Can you work these out from the model? Positions are in its coordinate system, mm. A direction names the side the tool comes from. Give positions to 0.01 mm unless a question says otherwise; leave off trailing zeros. Write each loop counter-clockwise with the first axis right and the second up, starting at its lowest first coordinate (ties: lowest second). Pieces come first, ordered by that corner, then holes. Notation, with made-up numbers: M 26,69.25 L 65,69.25 A20 cw 65,86.25 Z; hole C -7.5,38 d11. An arc over 180 degrees is marked long. Use CSV: the item, a comma, the result in double quotes. Start each with the question number.
from build123d import *

# Parameters (mm, degrees)
F1_DEPTH = 30
F3_D     = 3.5
F3_DEPTH = 5


with BuildPart() as f1:
    # F0 (on Front) → F1 (new body)
    with BuildSketch(Plane.XZ):
        Polygon((27.040993, 7.364779), (-2.959007, 7.364779), (-2.959007, -17.635221), (7.234091, -26.008121), (8.50357, -24.462669), (-0.959007, -16.689839), (-0.959007, 5.364779), (27.040993, 5.364779), align=None)
    extrude(amount=F1_DEPTH)

    # F3
    with Locations(Plane.XY.offset(7.364779)):
        with Locations((7.040993, -10), (17.040993, -15), (7.040993, -20)):
            Hole(F3_D / 2, depth=F3_DEPTH)


solid = f1.part
(1) I want a section at A-A (y = -20). Write out the boundary of the cut face in (x, z), and give its area (3 significant figures).
(2) Thinking about a two-plate mould opening in Y: for faces 4 (the face through (12, -15, 7.365)), 5 (the face through (-1.4, 0, -3.1)), 6 (the face through (-1.4, -30, -3.1)), 7 (the face through (7.269, -18.265, 6.351)), which applies, released by +Y, released by -Y, zero draft, split by the parting line, or undercut?
(3) I want a section at D-D (x = 22.5). Write out the boundary of the cut face in (y, z).
(4) Will these pins go through, and if not, where does the flat tip stop? pin 1 Ø6.5 at (y, z) = (-7.5, -8) entering from +X; pin 2 Ø5.5 at (x, y) = (17.04, -15) entering from -Z; pin 3 Ø10 at (x, z) = (9, -9) entering from -Y; pin 4 Ø4 at (x, y) = (9.5, -21.5) entering from -Z.
(5) I want a section at B-B (x = 17). Write out the boundary of the cut face in (y, z).
(6) Please list where these lines run through material, in increasing order: L1, parallel to Z at x = 19.75, y = -9.25; L2, parallel to X at y = -9.5, z = 3.5; L3, parallel to Z at x = -0.5, y = -13.75. Write a range as [from, to].
(7) Which directions (+Z, -Z, +X, -X, +Y, -Y) give clear straight access to the entire face, cutting with the end or side of a thin tool? Please do faces 1 (the face through (-0.959, -15, -6)), 2 (the face through (7.9, -14.8, -25.2)), 3 (the face through (7.269, -8.265, 6.351)).
(8) I want a section at C-C (y = -6.5). Write out the boundary of the cut face in (x, z), and give its area (3 significant figures).
Geometry results:
1,outline,"M -2.96,-17.64 L 7.23,-26.01 L 8.5,-24.46 L -0.96,-16.69 L -0.96,5.36 L 5.29,5.36 L 5.29,7.36 L -2.96,7.36 Z; M 8.79,5.36 L 27.04,5.36 L 27.04,7.36 L 8.79,7.36 Z"
1,area,"123 mm2"
2,face 4,"zero draft"
2,face 5,"released by +Y"
2,face 6,"released by -Y"
2,face 7,"undercut"
3,outline,"M -30,5.36 L 0,5.36 L 0,7.36 L -30,7.36 Z"
4,pin 1,"stops at x = -0.96"
4,pin 2,"stops at z = 5.36"
4,pin 3,"passes through"
4,pin 4,"stops at z = -25.68"
5,outline,"M -30,5.36 L -16.75,5.36 L -16.75,7.36 L -30,7.36 Z; M -13.25,5.36 L 0,5.36 L 0,7.36 L -13.25,7.36 Z"
6,L1,"z = [5.36, 7.36]"
6,L2,"x = [-2.96, -0.96]"
6,L3,"z = [-19.66, -17.07], [5.36, 7.36]"
7,face 1,"+X, +Y, -Y"
7,face 2,"-Z, +X, +Y, -Y"
7,face 3,"+Z"
8,outline,"M -2.96,-17.64 L 7.23,-26.01 L 8.5,-24.46 L -0.96,-16.69 L -0.96,5.36 L 27.04,5.36 L 27.04,7.36 L -2.96,7.36 Z"
8,area,"130 mm2"
